from build123d import *

# Parameters (mm, degrees)
F0_W     = 104.370906
F0_H     = 111.990906
F2_DEPTH = 25.4
F1_R     = 52.088044
F3_DEPTH = 50.8
F4_R     = 37.70573
F5_DEPTH = 50.801
F7_DEPTH = 17.78
F9_DEPTH = 60.288576


with BuildPart() as f2:
    # F0 (on Top) → F2 (new body)
    with BuildSketch(Plane.XY):
        Rectangle(F0_W, F0_H)
    extrude(amount=F2_DEPTH)

    # F1 (on Top) → F3 (join)
    with BuildSketch(Plane.XY):
        with Locations((-0.035915, -55.473275)):
            Circle(F1_R)
    extrude(amount=F3_DEPTH)

    # F4 (on face) → F5 (cut, through all)
    with BuildSketch(Plane.XY.offset(50.8)):
        with Locations((-0.035915, -55.473275)):
            Circle(F4_R)
    extrude(amount=-F5_DEPTH, mode=Mode.SUBTRACT)

    # F6 (on face) → F7 (join)
    with BuildSketch(Plane.XY.offset(25.4)):
        with BuildLine():
            ThreePointArc((-8.102123, -4.013576), (0.000443, -3.385244), (8.102123, -4.024887))
            Line((8.102123, -4.024887), (8.102123, 38.277184))
            Line((8.102123, 38.277184), (-8.102123, 38.277184))
            Line((-8.102123, 38.277184), (-8.102123, -4.013576))
        make_face()
    extrude(amount=F7_DEPTH)

    # F8 (on face) → F9 (cut, through all)
    with BuildSketch(Plane(origin=(-8.102123, 0, 0), x_dir=(0, -1, 0), z_dir=(-1, 0, 0))):
        Polygon((-38.277184, 43.18), (-38.277184, 25.4), (4.013576, 43.18), align=None)
    extrude(amount=-F9_DEPTH, mode=Mode.SUBTRACT)


solid = f2.part
For this review, take the finished solid that the model builds, in its own axes (mm). A direction names the side the tool comes from. Coordinates: 2 decimals unless noted, no trailing zeros. Order: outer loops, then holes, each group sorted by start corner. A loop starts at its lowest first (then second) coordinate and runs counter-clockwise, first axis right, second up. Notation, with made-up numbers: (-20.75, 70.5) - (-5.75, 70.5) arc R12 cw to (-5.75, 89.5) - close; hole circle Ø3 at (40.25, 38.25). An arc over 180 degrees is marked (long way). Use one line per item in the form item = value.
Q1. Consider section D-D (y = 40). Give the boundary of the cut face in (x, z), then the cut area to 3 significant figures.
Checked values:
outline = (-52.19, 0) - (52.19, 0) - (52.19, 25.4) - (-52.19, 25.4) - close
area = 2,650 mm2
Q2. Consider section A-A (y = -42). Give the boundary of the cut face in (x, z), then the cut area to 3 significant figures.
Checked values:
outline = (-52.19, 0) - (-35.25, 0) - (-35.25, 50.8) - (-50.35, 50.8) - (-50.35, 25.4) - (-52.19, 25.4) - close; (35.18, 0) - (52.19, 0) - (52.19, 25.4) - (50.28, 25.4) - (50.28, 50.8) - (35.18, 50.8) - close
area = 1,630 mm2
Q3. Consider section C-C (z = 33). Give the boundary of the cut face in (x, y), then the cut area to 3 significant figures.
Checked values:
outline = (-8.1, -4.01) arc R52.09 ccw (long way) to (8.1, -4.02) - (8.1, 20.2) - (-8.1, 20.2) - close; hole circle Ø75.41 at (-0.04, -55.47)
area = 4,440 mm2
Q4. For faces 5 (the flat face through (-1, 55.995, 13)), 6 (the flat face through (-12, 26, 25.4)), 7 (the flat face through (-8.102, 8, 30)), list the 3-axis set-ups (+Z, -Z, +X, -X, +Y, -Y) from which the entire face can be reached by the end or side of a thin tool; tool diameter is ignored.
Checked values:
face_5 = +Z, -Z, +X, -X, +Y
face_6 = +Z, +Y
face_7 = +Z, -X, +Y
Q5. For probe 1 along Y at (x, z) = (0, 19.5); probe 2 along Z at (x, y) = (41.5, -4); probe 3 along Y at (x, z) = (-19, 48), list the stretches that pass through material, from the lowest coordinate up. Write a range as from..to.
Checked values:
probe_1 = -107.56..-93.18, -17.77..56
probe_2 = 0..25.4
probe_3 = -103.99..-88.06, -22.88..-6.96
Q6. Draft analysis for pull direction X (two halves, no side actions). For faces 1 (the cylindrical face through (-4.944, -18.088, 25.756)), 2 (the flat face through (34.45, -39.8, 50.8)), 3 (the flat face through (8.102, 12, 32)), 4 (the cylindrical face through (-11.328, -106.323, 30.689)), state which applies: +X half, -X half, draft (parallel to the pull), parting line (faces both ways), or undercut.
Checked values:
face_1 = undercut
face_2 = draft
face_3 = +X half
face_4 = parting line
Q7. For P1, Ø1.5, axis at y = -80, z = 36, coming from the -X side; P2, Ø10, axis at x = -23, z = 35.5, coming from the +Y side; P3, Ø1, axis at y = -21, z = 30, coming from the -X side, all flat-tipped, find the tip position at first contact; note any pin that passes through.
Checked values:
P1 = -46.38
P2 = -6.58
P3 = -39.52
Q8. Consider section B-B (x = 20.5). Give the boundary of the cut face in (y, z), then the cut area to 3 significant figures.
Checked values:
outline = (-103.34, 0) - (-87.1, 0) - (-87.1, 50.8) - (-103.34, 50.8) - close; (-23.85, 0) - (56, 0) - (56, 25.4) - (-7.6, 25.4) - (-7.6, 50.8) - (-23.85, 50.8) - close
area = 3,270 mm2
